Can you work these out from the model? Positions are in its coordinate system, mm. Face numbers are marked on the shaded views. Coordinates: 2 decimals unless noted, no trailing zeros. Write each loop counter-clockwise with the first axis right and the second up, starting at its lowest first coordinate (ties: lowest second). Pieces come first, ordered by that corner, then holes. Notation, with made-up numbers: M 42,49.25 L 88,49.25 A27 ccw 88,76.25 Z; hole C 76,-34 d6. An arc over 180 degrees is marked long. Use one line per item in the form item = value. Start each with the question number.
```python
from build123d import *

# Parameters (mm, degrees)
SKETCH1_W           = 155
SKETCH1_H           = 127
BOSS_EXTRUDE1_DEPTH = 1
CUT_EXTRUDE1_DEPTH  = 0.5
SKETCH3_R           = 2.5
CUT_EXTRUDE2_DEPTH  = 0.1


with BuildPart() as part:
    # Sketch1 → Boss-Extrude1 (new body)
    with BuildSketch(Plane(origin=(0, 0, 0), x_dir=(1, 0, 0), z_dir=(0, 1, 0))):
        Rectangle(SKETCH1_W, SKETCH1_H)
    extrude(amount=BOSS_EXTRUDE1_DEPTH)

    # Sketch2 → Cut-Extrude1 (cut)
    with BuildSketch(Plane(origin=(0, 1, 0), x_dir=(1, 0, 0), z_dir=(0, 1, 0))):
        with BuildLine():
            Line((2.75, -14.745762103), (2.75, -51.798849897))
            Line((2.75, -51.798849897), (-2.75, -51.798849897))
            Line((-2.75, -51.798849897), (-2.75, -14.745762103))
            ThreePointArc((-2.75, -14.745762103), (-10.606601718, -10.606601718), (-14.745762103, -2.75))
            Line((-14.745762103, -2.75), (-50, -2.75))
            Line((-50, -2.75), (-50, 2.75))
            Line((-50, 2.75), (-14.745762103, 2.75))
            ThreePointArc((-14.745762103, 2.75), (-10.606601718, 10.606601718), (-2.75, 14.745762103))
            Line((-2.75, 14.745762103), (-2.75, 51.798849897))
            Line((-2.75, 51.798849897), (2.75, 51.798849897))
            Line((2.75, 51.798849897), (2.75, 14.745762103))
            ThreePointArc((2.75, 14.745762103), (10.606601718, 10.606601718), (14.745762103, 2.75))
            Line((14.745762103, 2.75), (50, 2.75))
            Line((50, 2.75), (50, -2.75))
            Line((50, -2.75), (14.745762103, -2.75))
            ThreePointArc((14.745762103, -2.75), (10.606601718, -10.606601718), (2.75, -14.745762103))
        make_face()
    extrude(amount=-CUT_EXTRUDE1_DEPTH, mode=Mode.SUBTRACT)

    # Sketch3 → Cut-Extrude2 (cut)
    with BuildSketch(Plane(origin=(0, 0.5, 0), x_dir=(1, 0, 0), z_dir=(0, 1, 0))):
        with Locations(Location((0, 0, 0), (0, 0, 270))):
            Circle(SKETCH3_R)
    extrude(amount=-CUT_EXTRUDE2_DEPTH, mode=Mode.SUBTRACT)


solid = part.part
```
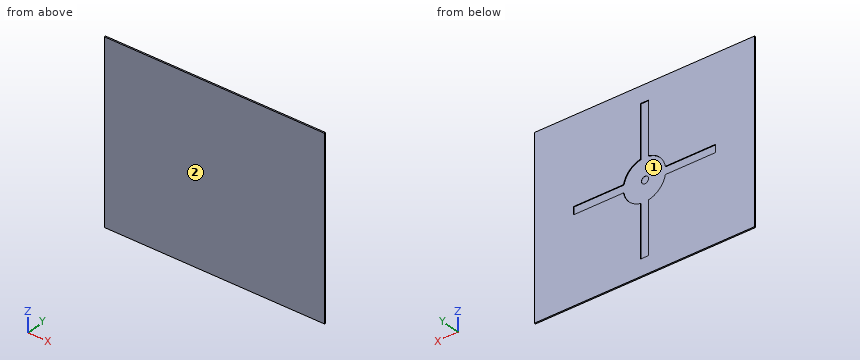
1) Please list where these lines run through material, in increasing order: line 1 (X direction, y = 0.85, z = -45.5); line 2 (X direction, y = 0.55, z = 0); line 3 (Y direction, x = -46.5, z = -2.5).
2) If we mould it in two halves opening along Z, with no side actions, what happens to the marked faces 1 and 2? For each: +Z half, -Z half, draft (parallel to the pull), parting line (faces both ways), or undercut.
3) Suppose I cut it at C-C on x = 0. Please give me the cut outline in (y, z).
4) Suppose I cut it at A-A on y = 0.8. Please give me the cut outline in (x, z).
5) Suppose I cut it at B-B on z = 0. Please give me the cut outline in (x, y).
6) Will these pins go through, and if not, where does the flat tip stop? pin 1 Ø4 at (x, z) = (-0.5, -1) entering from +Y; pin 2 Ø3 at (x, z) = (0, 0) entering from +Y; pin 3 Ø6 at (x, z) = (-33.5, -44.5) entering from -Y.
7) Suppose I cut it at D-D on z = 44. Please give me the cut outline in (x, y).
Computed values:
q1.line_1 = -77.5 to -2.75, 2.75 to 77.5
q1.line_2 = -77.5 to -50, 50 to 77.5
q1.line_3 = 0 to 0.5
q2.face_1 = undercut
q2.face_2 = draft
q3.outline = M 0,-63.5 L 1,-63.5 L 1,-51.8 L 0.5,-51.8 L 0.5,-2.5 L 0.4,-2.5 L 0.4,2.5 L 0.5,2.5 L 0.5,51.8 L 1,51.8 L 1,63.5 L 0,63.5 Z
q4.outline = M -77.5,-63.5 L 77.5,-63.5 L 77.5,63.5 L -77.5,63.5 Z; hole M -50,-2.75 L -14.75,-2.75 A15 ccw -2.75,-14.75 L -2.75,-51.8 L 2.75,-51.8 L 2.75,-14.75 A15 ccw 14.75,-2.75 L 50,-2.75 L 50,2.75 L 14.75,2.75 A15 ccw 2.75,14.75 L 2.75,51.8 L -2.75,51.8 L -2.75,14.75 A15 ccw -14.75,2.75 L -50,2.75 Z
q5.outline = M -77.5,0 L 77.5,0 L 77.5,1 L 50,1 L 50,0.5 L 2.5,0.5 L 2.5,0.4 L -2.5,0.4 L -2.5,0.5 L -50,0.5 L -50,1 L -77.5,1 Z
q6.pin_1 = 0.5
q6.pin_2 = 0.4
q6.pin_3 = 0
q7.outline = M -77.5,0 L 77.5,0 L 77.5,1 L 2.75,1 L 2.75,0.5 L -2.75,0.5 L -2.75,1 L -77.5,1 Z
